from build123d import *

# Parameters (mm, degrees)
SKETCH1_W           = 250
SKETCH1_H           = 45
BOSS_EXTRUDE1_DEPTH = 3.175
SKETCH4_R           = 3
SKETCH4_R_2         = 1.75
CUT_EXTRUDE1_DEPTH  = 227.144490592
SKETCH5_R           = 4.25
CUT_EXTRUDE2_DEPTH  = 227.144490592
SKETCH10_R          = 1.75
CUT_EXTRUDE4_DEPTH  = 227.144490592
FILLET1_R           = 7
SKETCH11_R          = 2.875
CUT_EXTRUDE5_DEPTH  = 227.144490592
SKETCH12_R          = 1.75
CUT_EXTRUDE6_DEPTH  = 227.144490592


with BuildPart() as part:
    # Sketch1 → Boss-Extrude1 (new body)
    with BuildSketch(Plane(origin=(0, 0, 0), x_dir=(1, 0, 0), z_dir=(0, 1, 0))):
        with Locations((100, 0)):
            Rectangle(SKETCH1_W, SKETCH1_H)
    extrude(amount=BOSS_EXTRUDE1_DEPTH)

    # Sketch4 → Cut-Extrude1 (cut, through all)
    with BuildSketch(Plane(origin=(0, 3.175, 0), x_dir=(1, 0, 0), z_dir=(0, 1, 0))):
        with Locations(Location((200, 0, 0), (0, 0, 270))):
            Circle(SKETCH4_R)
        with Locations(Location((186, 9, 0), (0, 0, 270))):
            Circle(SKETCH4_R_2)
        with Locations(Location((214, 9, 0), (0, 0, 90))):
            Circle(SKETCH4_R_2)
        with Locations(Location((214, -9, 0), (0, 0, 270))):
            Circle(SKETCH4_R_2)
        with Locations(Location((186, -9, 0), (0, 0, 90))):
            Circle(SKETCH4_R_2)
    extrude(amount=-CUT_EXTRUDE1_DEPTH, mode=Mode.SUBTRACT)

    # Sketch5 → Cut-Extrude2 (cut, through all)
    with BuildSketch(Plane(origin=(0, 3.175, 0), x_dir=(1, 0, 0), z_dir=(0, 1, 0))):
        with Locations(Location((0, 0, 0), (0, 0, 270))):
            Circle(SKETCH5_R)
    extrude(amount=-CUT_EXTRUDE2_DEPTH, mode=Mode.SUBTRACT)

    # Sketch10 → Cut-Extrude4 (cut, through all)
    with BuildSketch(Plane(origin=(0, 3.175, 0), x_dir=(1, 0, 0), z_dir=(0, 1, 0))):
        with Locations(Location((80.5, -17.5, 0), (0, 0, 270))):
            Circle(SKETCH10_R)
        with Locations(Location((166, -17.5, 0), (0, 0, 270))):
            Circle(SKETCH10_R)
        with Locations(Location((166, 17.5, 0), (0, 0, 90))):
            Circle(SKETCH10_R)
        with Locations(Location((80.5, 17.5, 0), (0, 0, 90))):
            Circle(SKETCH10_R)
        with Locations(Location((123.25, -17.5, 0), (0, 0, 270))):
            Circle(SKETCH10_R)
        with Locations(Location((123.25, 17.5, 0), (0, 0, 90))):
            Circle(SKETCH10_R)
    extrude(amount=-CUT_EXTRUDE4_DEPTH, mode=Mode.SUBTRACT)

    # Fillet1
    fillet1_edges = [part.edges().sort_by_distance(p)[0] for p in [
        (-25, 1.5875, -22.5),
        (225, 1.5875, -22.5),
        (225, 1.5875, 22.5),
        (-25, 1.5875, 22.5),
    ]]
    fillet(fillet1_edges, radius=FILLET1_R)

    # Sketch11 → Cut-Extrude5 (cut, through all)
    with BuildSketch(Plane(origin=(0, 3.175, 0), x_dir=(1, 0, 0), z_dir=(0, 1, 0))):
        with Locations(Location((0, 17.5, 0), (0, 0, 270))):
            Circle(SKETCH11_R)
        with Locations(Location((17.5, 0, 0), (0, 0, 270))):
            Circle(SKETCH11_R)
        with Locations(Location((0, -17.5, 0), (0, 0, 270))):
            Circle(SKETCH11_R)
        with Locations(Location((-17.5, 0, 0), (0, 0, 270))):
            Circle(SKETCH11_R)
    extrude(amount=-CUT_EXTRUDE5_DEPTH, mode=Mode.SUBTRACT)

    # Sketch12 → Cut-Extrude6 (cut, through all)
    with BuildSketch(Plane(origin=(0, 3.175, 0), x_dir=(1, 0, 0), z_dir=(0, 1, 0))):
        with Locations(Location((0, 8, 0), (0, 0, 270))):
            Circle(SKETCH12_R)
        with Locations(Location((8, 0, 0), (0, 0, 270))):
            Circle(SKETCH12_R)
        with Locations(Location((0, -8, 0), (0, 0, 270))):
            Circle(SKETCH12_R)
        with Locations(Location((-8, 0, 0), (0, 0, 270))):
            Circle(SKETCH12_R)
    extrude(amount=-CUT_EXTRUDE6_DEPTH, mode=Mode.SUBTRACT)


solid = part.part
Could you check a few things on this model? Use its own coordinates, in mm. Round coordinates to 2 decimals unless told otherwise and drop trailing zeros. Order: outer loops, then holes, each group sorted by start corner. A loop starts at its lowest first (then second) coordinate and runs counter-clockwise, first axis right, second up.
Q1. Please list where these lines run through material, in increasing order: probe 1 along Z at (x, y) = (214, 1.7); probe 2 along X at (y, z) = (0.8, -8); probe 3 along X at (y, z) = (1.6, -9).
Geometry says:
probe 1: z = -22.5 to -10.75, -7.25 to 7.25, 10.75 to 22.5
probe 2: x = -25 to -1.75, 1.75 to 184.56, 187.44 to 212.56, 215.44 to 225
probe 3: x = -25 to -1.44, 1.44 to 184.25, 187.75 to 212.25, 215.75 to 225
Q2. Imagine slicing it at A-A, the plane x = 200. List the corners of the cut face in (y, z) for me (3 decimals).
Geometry says:
outline: (0, -22.5) - (3.175, -22.5) - (3.175, -3) - (0, -3) - close; (0, 3) - (3.175, 3) - (3.175, 22.5) - (0, 22.5) - close
Q3. Imagine slicing it at C-C, the plane x = 17.5. List the corners of the cut face in (y, z) for me (3 decimals).
Geometry says:
outline: (0, -22.5) - (3.175, -22.5) - (3.175, -2.875) - (0, -2.875) - close; (0, 2.875) - (3.175, 2.875) - (3.175, 22.5) - (0, 22.5) - close
Q4. Imagine slicing it at B-B, the plane y = 2.25. State how many separate pieces and enclosed holes the cut face has, then the cut area to 3 significant figures.
Geometry says:
separate pieces: 1
enclosed holes: 20
area: 10,900 mm2
